For this review, take the finished solid that the model builds, in its own axes (mm). A direction names the side the tool comes from. Coordinates: 2 decimals unless noted, no trailing zeros. Write each loop counter-clockwise with the first axis right and the second up, starting at its lowest first coordinate (ties: lowest second). Pieces come first, ordered by that corner, then holes.
```python
from build123d import *

# Parameters (mm, degrees)
SCHIZZO2_R                   = 25
SCHIZZO2_R_2                 = 17.5
ESTRUSIONE_ESTRUSIONE1_DEPTH = 4
SCHIZZO3_R                   = 1.6
ESTRUSIONE_ESTRUSIONE2_DEPTH = 2
RIPETIZIONECIRCOLARE1_COUNT  = 3


with BuildPart() as part:
    # Schizzo2 → Estrusione-Estrusione1 (new body)
    with BuildSketch(Plane.XY):
        Circle(SCHIZZO2_R)
        Circle(SCHIZZO2_R_2, mode=Mode.SUBTRACT)
    extrude(amount=ESTRUSIONE_ESTRUSIONE1_DEPTH)

    # Schizzo3 → Estrusione-Estrusione2 (add)
    with BuildSketch(Plane(origin=(-0.75, 1.299038106, 0), x_dir=(0, 0, -1), z_dir=(-0.5000000000000043, 0.866025403784436, 0))):
        with BuildLine():
            Line((-11.341531907, -14.184207936), (-4, -17.5))
            Line((-4, -17.5), (-4, -25))
            Line((-4, -25), (-10.523132314, -20.868682868))
            ThreePointArc((-10.523132314, -20.868682868), (-12.223574858, -19.90479517), (-14.009986273, -19.111499134))
            ThreePointArc((-14.009986273, -19.111499134), (-15.569198234, -15.386797217), (-11.785347493, -13.977180291))
            ThreePointArc((-11.785347493, -13.977180291), (-11.564073393, -14.082052593), (-11.341531907, -14.184207936))
        make_face()
        with Locations(Location((-13, -16.5, 0), (0, 0, 270))):
            Circle(SCHIZZO3_R, mode=Mode.SUBTRACT)
    estrusione_estrusione2 = extrude(amount=ESTRUSIONE_ESTRUSIONE2_DEPTH)

    # RipetizioneCircolare1: Estrusione-Estrusione2 ×3 about axis
    ripetizionecircolare1_axis = Axis((0, 0, 0), (0, 0, 1))
    for i in range(1, RIPETIZIONECIRCOLARE1_COUNT):
        add(estrusione_estrusione2.rotate(ripetizionecircolare1_axis, i * 360 / RIPETIZIONECIRCOLARE1_COUNT))


solid = part.part
```
Q1. Add section D-D (y = -16.5). State the section outline as (x, z) points, then the cut area to 3 significant figures.
Ans:
outline: (-18.78, 0) - (-5.83, 0) - (-5.83, 4) - (-18.78, 4) - close; (1.5, 6.21) - (3.5, 6.21) - (3.5, 11.4) - (1.5, 11.4) - close; (1.5, 14.6) - (3.5, 14.6) - (3.5, 15.8) - (1.5, 15.8) - close; (5.83, 0) - (18.78, 0) - (18.78, 4) - (5.83, 4) - close
area: 116 mm2
Q2. Tool access review of faces 1 (the flat face through (14.939, 12.667, 8.506)), 2 (the flat face through (1.5, -19, 9)), 3 (the flat face through (-17.439, 8.336, 8.506)), 4 (the flat face through (-18.439, 6.604, 8.506)): name each direction out of +Z, -Z, +X, -X, +Y, -Y from which nothing blocks a thin tool from reaching the whole face with its end or side.
Ans:
face 1: +Z, -X, +Y
face 2: +Z, -X, +Y, -Y
face 3: +Z, +Y
face 4: +Z, -X, -Y
Q3. Add section C-C (z = 5.5). State the section outline as (x, y) points.
Ans:
outline: (-22.58, 8.99) - (-16.32, 5.38) - (-15.32, 7.11) - (-21.58, 10.73) - close; (1.5, -24.05) - (3.5, -24.05) - (3.5, -16.82) - (1.5, -16.82) - close; (12.82, 11.44) - (13.82, 9.71) - (20.08, 13.32) - (19.08, 15.06) - close
Q4. Clearance check with flat-ended pins moving along their axes: pin 1 Ø9 at (y, z) = (-22, 9.5) entering from +X; pin 2 Ø12 at (x, y) = (-1.5, -9.5) entering from +Z; pin 3 Ø8 at (x, z) = (16, 2) entering from -Y. State where each tip first meets the part, or that it passes through.
Ans:
pin 1: stops at x = 3.5
pin 2: stops at z = 15.14
pin 3: stops at y = -21.93
Q5. For probe 1 along Y at (x, z) = (0, 1.95); probe 2 along Z at (x, y) = (-18, -11.5); probe 3 along X at (y, z) = (-16.5, 9.75), list the stretches that pass through material, from the lowest coordinate up.
Ans:
probe 1: y = -25 to -17.5, 17.5 to 25
probe 2: z = 0 to 4
probe 3: x = 1.5 to 3.5
Q6. Draft analysis for pull direction Z (two halves, no side actions). For faces 5 (the flat face through (2.49, -22.96, 7.22)), 6 (the flat face through (15.939, 10.934, 8.506)), 7 (the cylindrical face through (14.368, 11.166, 12.519)), 8 (the cylindrical face through (-14.43, 5.46, 13.97)), state which applies: +Z half, -Z half, draft (parallel to the pull), parting line (faces both ways), or undercut.
Ans:
face 5: +Z half
face 6: draft
face 7: undercut
face 8: undercut
Q7. Add section A-A (y = 0). State the section outline as (x, z) points, then the cut area to 3 significant figures.
Ans:
outline: (-25, 0) - (-17.5, 0) - (-17.5, 4) - (-25, 4) - close; (17.5, 0) - (25, 0) - (25, 4) - (17.5, 4) - close
area: 60.0 mm2
